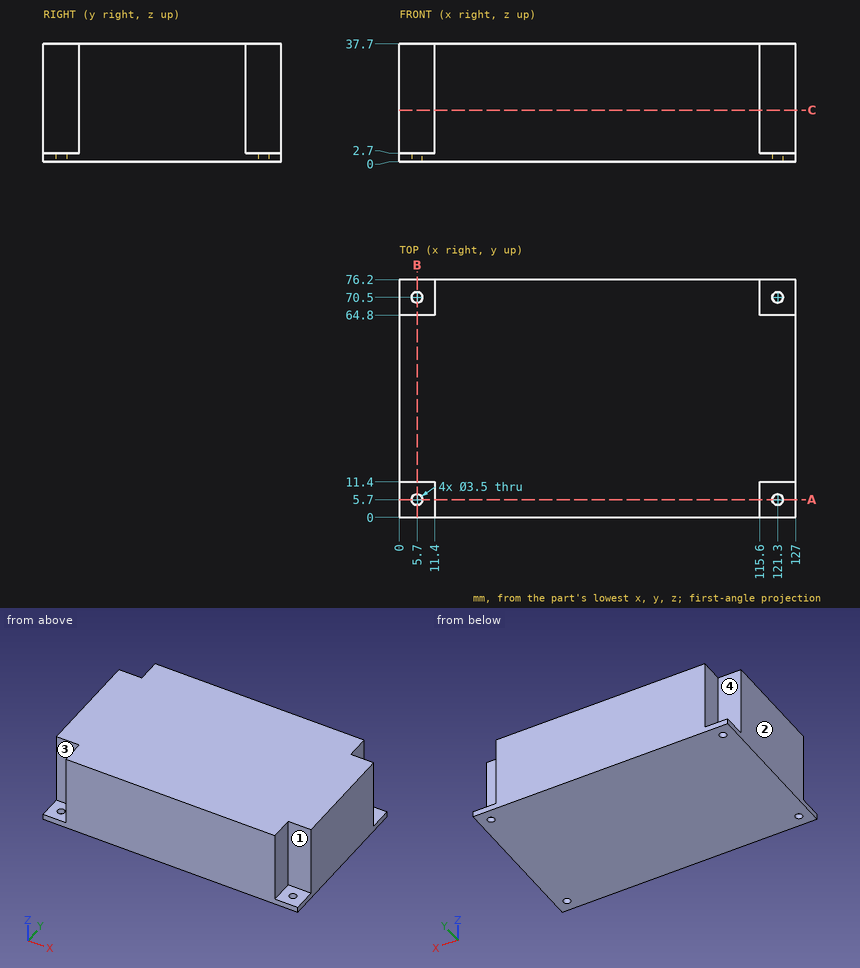
Design review of the part shown in the three views and the two pictorial views. Dimensions are in mm from the part's minimum x, y and z. A direction names the side the tool comes from. Round coordinates to 2 decimals unless told otherwise and drop trailing zeros. Write each loop counter-clockwise with the first axis right and the second up, starting at its lowest first coordinate (ties: lowest second). Pieces come first, ordered by that corner, then holes. Notation, with made-up numbers: M -20.5,-11 L 6.5,-11 A23 ccw 6.5,20 Z; hole C 76,-3 d9. An arc over 180 degrees is marked long. One line per item, written item: value. Start each with the question number.
1. Take a section at B-B on x = 5.7. State the section outline as (y, z) points.
2. For the marked faces 1, 2, 3 and 4, list the 3-axis set-ups (+Z, -Z, +X, -X, +Y, -Y) from which the entire face can be reached by the end or side of a thin tool; tool diameter is ignored.
3. Take a section at C-C on z = 16.5. State the section outline as (x, y) points.
4. Take a section at A-A on y = 5.7. State the section outline as (x, z) points.
5. To check wall thickness, follow probe 1 along X at (y, z) = (70.5, 2.05); probe 2 along Y at (x, z) = (5.7, 2); probe 3 along X at (y, z) = (5, 1). State the ranges of each line that lie inside material, in increasing order. Write a range as from..to.
6. Clearance check with flat-ended pins moving along their axes: P1, Ø9, axis at x = 122.5, z = 29, coming from the +Y side; P2, Ø4, axis at x = 5.7, y = 5.7, coming from the +Z side; P3, Ø4.5, axis at x = 5.7, y = 70.5, coming from the -Z side; P4, Ø12.5, axis at x = 122, z = 27.5, coming from the -Y side. State where each tip first meets the part, or that it passes through.
Computed:
1. outline: M 0,0 L 3.95,0 L 3.95,2.7 L 0,2.7 Z; M 7.45,0 L 68.75,0 L 68.75,2.7 L 64.8,2.7 L 64.8,37.7 L 11.4,37.7 L 11.4,2.7 L 7.45,2.7 Z; M 72.25,0 L 76.2,0 L 76.2,2.7 L 72.25,2.7 Z
2. face 1: +Z, +X, -Y
2. face 2: +Z, -Z, -X, +Y, -Y
2. face 3: +Z, -X, -Y
2. face 4: +Z, -X, +Y
3. outline: M 0,11.4 L 11.4,11.4 L 11.4,0 L 115.6,0 L 115.6,11.4 L 127,11.4 L 127,64.8 L 115.6,64.8 L 115.6,76.2 L 11.4,76.2 L 11.4,64.8 L 0,64.8 Z
4. outline: M 0,0 L 3.95,0 L 3.95,2.7 L 0,2.7 Z; M 7.45,0 L 119.55,0 L 119.55,2.7 L 115.6,2.7 L 115.6,37.7 L 11.4,37.7 L 11.4,2.7 L 7.45,2.7 Z; M 123.05,0 L 127,0 L 127,2.7 L 123.05,2.7 Z
5. probe 1: x = 0..3.95, 7.45..119.55, 123.05..127
5. probe 2: y = 0..3.95, 7.45..68.75, 72.25..76.2
5. probe 3: x = 0..4.1, 7.3..119.7, 122.9..127
6. P1: stops at y = 64.8
6. P2: stops at z = 2.7
6. P3: stops at z = 0
6. P4: stops at y = 11.4
